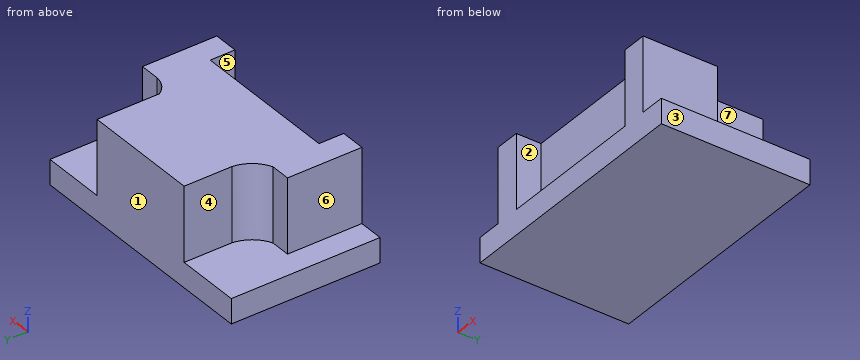
```python
from build123d import *

# Parameters (mm, degrees)
F0_W      = 63.5
F0_H      = 38.1
F1_DEPTH  = 6.35
F2_W      = 50.8
F2_H      = 38.1
F3_DEPTH  = 19.05
F4_W      = 38.1
F4_H      = 6.35
F5_DEPTH  = 19.05
F6_W      = 10.16
F6_H      = 19.05
F7_DEPTH  = 19.05
F8_DEPTH  = 19.05
F10_DEPTH = 19.05
F12_DEPTH = 19.05


with BuildPart() as f1:
    # F0 (on Top) → F1 (new body)
    with BuildSketch(Plane.XY):
        Rectangle(F0_W, F0_H)
    extrude(amount=F1_DEPTH)

    # F2 (on face) → F3 (join)
    with BuildSketch(Plane.XY.offset(6.35)):
        Rectangle(F2_W, F2_H)
    extrude(amount=F3_DEPTH)

    # F4 (on face) → F5 (cut)
    with BuildSketch(Plane.XY.offset(25.4)):
        with Locations((0, -15.875)):
            Rectangle(F4_W, F4_H)
    extrude(amount=-F5_DEPTH, mode=Mode.SUBTRACT)

    # F6 (on face) → F7 (cut)
    with BuildSketch(Plane.XY.offset(25.4)):
        with Locations((-20.32, 9.525)):
            Rectangle(F6_W, F6_H)
    extrude(amount=-F7_DEPTH, mode=Mode.SUBTRACT)

    # F6 (on face) → F8 (cut)
    with BuildSketch(Plane.XY.offset(25.4)):
        with Locations((20.32, 9.525)):
            Rectangle(F6_W, F6_H)
    extrude(amount=-F8_DEPTH, mode=Mode.SUBTRACT)

    # F9 (on face) → F10 (join)
    with BuildSketch(Plane.XY.offset(6.35)):
        with BuildLine():
            ThreePointArc((-15.24, 6.8340138532), (-16.8394418456, 2.717851858), (-20.32, 0))
            Line((-20.32, 0), (-15.24, 0))
            Line((-15.24, 0), (-15.24, 6.8340138532))
        make_face()
    extrude(amount=F10_DEPTH)

    # F11 (on face) → F12 (join)
    with BuildSketch(Plane.XY.offset(6.35)):
        with BuildLine():
            ThreePointArc((20.32, 0), (17.3902858448, 0.9238566208), (15.24, 3.1177132417))
            Line((15.24, 3.1177132417), (15.24, 0))
            Line((15.24, 0), (20.32, 0))
        make_face()
    extrude(amount=F12_DEPTH)


solid = f1.part
```
The listing builds one solid part. Answer for the finished solid, in the listing's coordinates (mm). Face numbers are marked on the shaded views. A direction names the side the tool comes from. Coordinates: 2 decimals unless noted, no trailing zeros. Write each loop counter-clockwise with the first axis right and the second up, starting at its lowest first coordinate (ties: lowest second). Pieces come first, ordered by that corner, then holes.
Q1. Section D-D, the plane y = -10.5 is taken. Write down the section's boundary in (x, z), then the cut area to 3 significant figures.
Returned:
outline: (-31.75, 0) - (31.75, 0) - (31.75, 6.35) - (25.4, 6.35) - (25.4, 25.4) - (-25.4, 25.4) - (-25.4, 6.35) - (-31.75, 6.35) - close
area: 1,370 mm2
Q2. The mould has two halves that part along X. Classify the marked faces 1, 2, 3 and 4: released by +X, released by -X, zero draft, split by the parting line, or undercut.
Returned:
face 1: zero draft
face 2: undercut
face 3: released by +X
face 4: released by -X
Q3. Find the intervals of material crossed by line 1 along X through (y, z) = (-16, 7.25); line 2 along Y through (x, z) = (10, 23.75); line 3 along X through (y, z) = (-6, 23.75), in increasing order.
Returned:
line 1: x = -25.4 to -19.05, 19.05 to 25.4
line 2: y = -12.7 to 19.05
line 3: x = -25.4 to 25.4
Q4. Section C-C, the plane x = -10.5 is taken. Write down the section's boundary in (y, z), then the cut area to 3 significant figures.
Returned:
outline: (-19.05, 0) - (19.05, 0) - (19.05, 25.4) - (-12.7, 25.4) - (-12.7, 6.35) - (-19.05, 6.35) - close
area: 847 mm2
Q5. Given P1, Ø2, axis at x = -3.5, z = 15, coming from the -Y side; P2, Ø5, axis at x = -8, y = -15.5, coming from the +Z side; P3, Ø5, axis at y = 11, z = 11.5, coming from the +X side, each flat-ended and moving along its own axis, determine where each tip first touches the part or whether it passes through.
Returned:
P1: stops at y = -12.7
P2: stops at z = 6.35
P3: stops at x = 15.24
Q6. Section B-B, the plane y = 16 is taken. Write down the section's boundary in (x, z), then the cut area to 3 significant figures.
Returned:
outline: (-31.75, 0) - (31.75, 0) - (31.75, 6.35) - (15.24, 6.35) - (15.24, 25.4) - (-15.24, 25.4) - (-15.24, 6.35) - (-31.75, 6.35) - close
area: 984 mm2
Q7. Which of the six approach directions +Z, -Z, +X, -X, +Y, -Y give full straight-line access (tool end or side, diameter ignored) to the marked faces 5, 6 and 7?
Returned:
face 5: +Z, -Y
face 6: +Z, -X, +Y, -Y
face 7: +Z, +X, +Y
Q8. Section A-A, the plane z = 15.25 is taken. Write down the section's boundary in (x, y), then the cut area to 3 significant figures.
Returned:
outline: (-25.4, -19.05) - (-19.05, -19.05) - (-19.05, -12.7) - (19.05, -12.7) - (19.05, -19.05) - (25.4, -19.05) - (25.4, 0) - (20.32, 0) arc R6.33 cw to (15.24, 3.12) - (15.24, 19.05) - (-15.24, 19.05) - (-15.24, 6.83) arc R8.32 cw to (-20.32, 0) - (-25.4, 0) - close
area: 1,320 mm2
